Study the drawing (mm; zero at the part's minimum x, y, z) and answer. Round coordinates to 2 decimals unless told otherwise and drop trailing zeros. Order: outer loops, then holes, each group sorted by start corner. A loop starts at its lowest first (then second) coordinate and runs counter-clockwise, first axis right, second up. Notation, with made-up numbers: (48.25, -21) - (55.25, -21) arc R23 cw to (55.25, -3) - close; hole circle Ø9 at (54.5, 79). An arc over 180 degrees is marked (long way). Use one line per item in the form item = value. Start each with the question number.
Q1. The part is cut by section C-C on x = 22.6. Determine the outline of the cut face in (y, z), plus the area to 3 significant figures.
Q2. The part is cut by section A-A on y = 2.15. State how many separate pieces and enclosed holes the cut face has, plus the area to 3 significant figures.
Q3. Find the intervals of material crossed by line 1 (Z direction, x = 22.6, y = 1.75); line 2 (Z direction, x = 52.5, y = 0.85); line 3 (X direction, y = 1.45, z = 54), in increasing order. Write a range as [from, to].
Q4. The part is cut by section D-D on z = 45. Determine the outline of the cut face in (x, y), plus the area to 3 significant figures.
Q5. The part is cut by section B-B on x = 44. Determine the outline of the cut face in (y, z).
Q6. Given P1, Ø1.5, axis at x = 32.5, z = 39.5, coming from the -Y side; P2, Ø0.9, axis at y = 1, z = 59, coming from the +X side; P3, Ø1.5, axis at x = 79.5, y = 1.5, coming from the +Z side; P4, Ø0.9, axis at y = 1, z = 2, coming from the +X side, each flat-ended and moving along its own axis, determine where each tip first touches the part or whether it passes through.
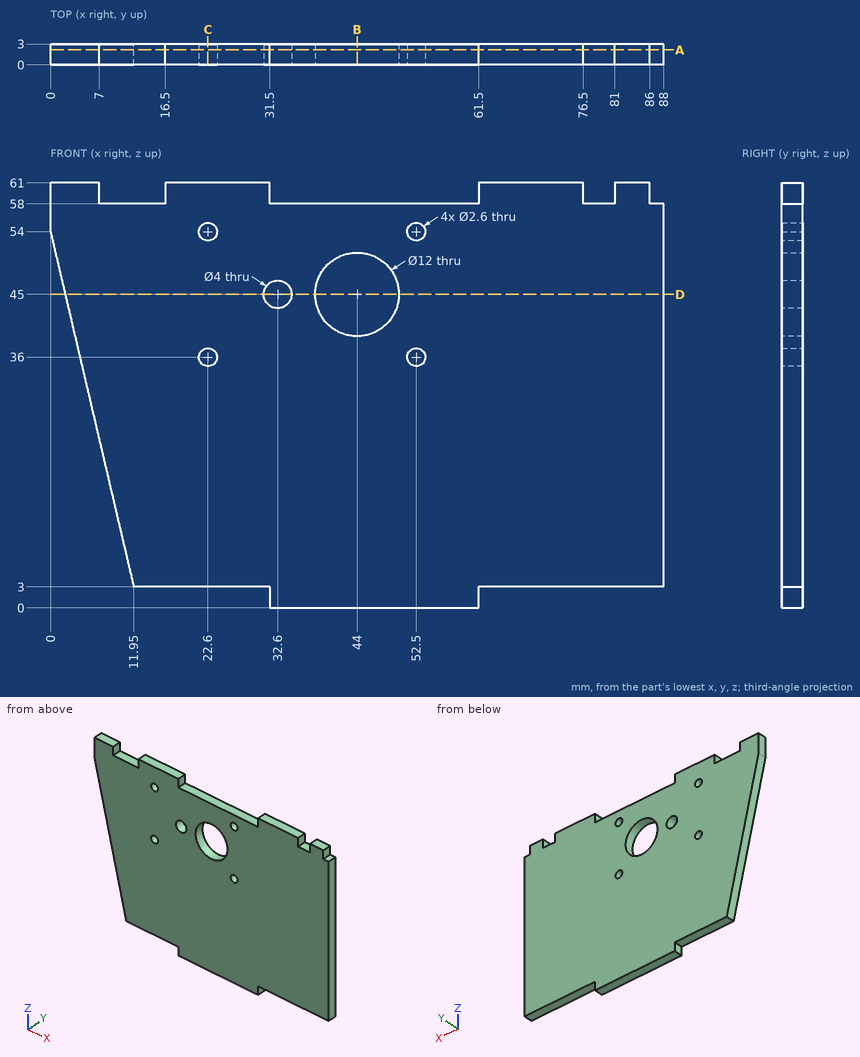
Found:
q1.outline = (0, 3) - (3, 3) - (3, 34.7) - (0, 34.7) - close; (0, 37.3) - (3, 37.3) - (3, 52.7) - (0, 52.7) - close; (0, 55.3) - (3, 55.3) - (3, 61) - (0, 61) - close
q1.area = 158 mm²
q2.separate_pieces = 1
q2.enclosed_holes = 6
q2.area = 4,600 mm²
q3.line_1 = [3, 34.7], [37.3, 52.7], [55.3, 61]
q3.line_2 = [0, 34.7], [37.3, 52.7], [55.3, 58]
q3.line_3 = [0, 21.3], [23.9, 51.2], [53.8, 88]
q4.outline = (2.11, 0) - (30.6, 0) - (30.6, 3) - (2.11, 3) - close; (34.6, 0) - (38, 0) - (38, 3) - (34.6, 3) - close; (50, 0) - (88, 0) - (88, 3) - (50, 3) - close
q4.area = 210 mm²
q5.outline = (0, 0) - (3, 0) - (3, 39) - (0, 39) - close; (0, 51) - (3, 51) - (3, 58) - (0, 58) - close
q6.P1 = 0
q6.P2 = 86
q6.P3 = 58
q6.P4 = 61.5
